The listing builds one solid part. Answer for the finished solid, in the listing's coordinates (mm). Give positions to 0.01 mm unless a question says otherwise; leave off trailing zeros. Loops run counter-clockwise (first coordinate to the right, second up) from the corner with the lowest first, then second, coordinate; pieces in that order, holes last. Notation, with made-up numbers: M 57,31 L 74,31 A12 ccw 74,54 Z; hole C -1,-36.75 d2. An arc over 180 degrees is marked long. Use one line per item in the form item = value. Start each with the question number.
1. The mould has two halves that part along Z. Classify faces 1 (the face through (46.97, 1.61, 41.86)), 2 (the face through (-1, 2, -43)), 3 (the face through (-1, 0, -1)), 4 (the face through (-40.674, 1.565, 22.616)): released by +Z, released by -Z, zero draft, split by the parting line, or undercut.
2. The part is cut by section C-C (z = -19). Give the number of separate pieces and of enclosed holes in the cut face, and give its area (3 significant figures).
3. The part is cut by section B-B (x = 24). Write down the section's boundary in (y, z) (3 decimals).
4. The part is cut by section A-A (z = -35). Write down the section's boundary in (x, y) (3 decimals).
5. Straight lines are drawn through the part: line 1 (X direction, y = 1.05, z = -35) (3 decimals); line 2 (X direction, y = 2.6, z = -25) (3 decimals); line 3 (X direction, y = 1.45, z = -22.5) (3 decimals). For each, find the intervals that lie inside material, in ascending order. Write a range as from..to.
6. Each of these flat-tipped pins is pushed along its axis until it touches: pin 1 Ø2.5 at (x, z) = (-42.68, -18.67) entering from +Y; pin 2 Ø6.5 at (x, z) = (-42.68, 5.84) entering from +Y (3 decimals). Where does it stop, or does it pass through?
from build123d import *

# Parameters (mm, degrees)
SKETCH1_W           = 96.35
SKETCH1_H           = 86
SKETCH1_R           = 2.05
BOSS_EXTRUDE1_DEPTH = 3.175
FILLET1_R           = 4
SKETCH2_R           = 7.05
CUT_EXTRUDE1_DEPTH  = 3.18


with BuildPart() as part:
    # Sketch1 → Boss-Extrude1 (new body)
    with BuildSketch(Plane(origin=(0, 0, 0), x_dir=(1, 0, 0), z_dir=(0, 1, 0))):
        Rectangle(SKETCH1_W, SKETCH1_H)
        with Locations(Location((42.675, 35, 0), (0, 0, 270))):
            Circle(SKETCH1_R, mode=Mode.SUBTRACT)
        with Locations(Location((42.675, 26.832661921, 0), (0, 0, 270))):
            Circle(SKETCH1_R, mode=Mode.SUBTRACT)
        with Locations(Location((42.675, 18.665323842, 0), (0, 0, 270))):
            Circle(SKETCH1_R, mode=Mode.SUBTRACT)
        with Locations(Location((42.675, 10.497985763, 0), (0, 0, 270))):
            Circle(SKETCH1_R, mode=Mode.SUBTRACT)
        with Locations(Location((42.675, 2.330647684, 0), (0, 0, 270))):
            Circle(SKETCH1_R, mode=Mode.SUBTRACT)
        with Locations(Location((42.675, -5.836690395, 0), (0, 0, 270))):
            Circle(SKETCH1_R, mode=Mode.SUBTRACT)
        with Locations(Location((42.675, -14.004028475, 0), (0, 0, 270))):
            Circle(SKETCH1_R, mode=Mode.SUBTRACT)
        with Locations(Location((42.675, -22.171366554, 0), (0, 0, 270))):
            Circle(SKETCH1_R, mode=Mode.SUBTRACT)
        with Locations(Location((42.675, -30.338704633, 0), (0, 0, 270))):
            Circle(SKETCH1_R, mode=Mode.SUBTRACT)
        with Locations(Location((42.675, -38.506042712, 0), (0, 0, 270))):
            Circle(SKETCH1_R, mode=Mode.SUBTRACT)
        with Locations(Location((-42.675, -38.506042712, 0), (0, 0, 90))):
            Circle(SKETCH1_R, mode=Mode.SUBTRACT)
        with Locations(Location((-42.675, -30.338704633, 0), (0, 0, 90))):
            Circle(SKETCH1_R, mode=Mode.SUBTRACT)
        with Locations(Location((-42.675, -22.171366554, 0), (0, 0, 90))):
            Circle(SKETCH1_R, mode=Mode.SUBTRACT)
        with Locations(Location((-42.675, -14.004028475, 0), (0, 0, 90))):
            Circle(SKETCH1_R, mode=Mode.SUBTRACT)
        with Locations(Location((-42.675, -5.836690395, 0), (0, 0, 90))):
            Circle(SKETCH1_R, mode=Mode.SUBTRACT)
        with Locations(Location((-42.675, 2.330647684, 0), (0, 0, 90))):
            Circle(SKETCH1_R, mode=Mode.SUBTRACT)
        with Locations(Location((-42.675, 10.497985763, 0), (0, 0, 90))):
            Circle(SKETCH1_R, mode=Mode.SUBTRACT)
        with Locations(Location((-42.675, 18.665323842, 0), (0, 0, 90))):
            Circle(SKETCH1_R, mode=Mode.SUBTRACT)
        with Locations(Location((-42.675, 26.832661921, 0), (0, 0, 90))):
            Circle(SKETCH1_R, mode=Mode.SUBTRACT)
        with Locations(Location((-42.675, 35, 0), (0, 0, 90))):
            Circle(SKETCH1_R, mode=Mode.SUBTRACT)
    extrude(amount=BOSS_EXTRUDE1_DEPTH)

    # Fillet1
    fillet1_edges = [part.edges().sort_by_distance(p)[0] for p in [
        (48.175, 1.5875, 43),
        (-48.175, 1.5875, 43),
        (-48.175, 1.5875, -43),
        (48.175, 1.5875, -43),
    ]]
    fillet(fillet1_edges, radius=FILLET1_R)

    # Sketch2 → Cut-Extrude1 (cut)
    with BuildSketch(Plane(origin=(0, 3.175, 0), x_dir=(1, 0, 0), z_dir=(0, 1, 0))):
        with Locations(Location((-24, 19, 0), (0, 0, 270))):
            Circle(SKETCH2_R)
        with Locations(Location((24, 19, 0), (0, 0, 270))):
            Circle(SKETCH2_R)
    extrude(amount=-CUT_EXTRUDE1_DEPTH, mode=Mode.SUBTRACT)


solid = part.part
Derived:
q1.face_1 = released by +Z
q1.face_2 = released by -Z
q1.face_3 = zero draft
q1.face_4 = undercut
q2.separate_pieces = 5
q2.enclosed_holes = 0
q2.area = 191 mm2
q3.outline = M 0,-43 L 3.175,-43 L 3.175,-26.05 L 0,-26.05 Z; M 0,-11.95 L 3.175,-11.95 L 3.175,43 L 0,43 Z
q4.outline = M -48.175,0 L -44.725,0 L -44.725,3.175 L -48.175,3.175 Z; M -40.625,0 L 40.625,0 L 40.625,3.175 L -40.625,3.175 Z; M 44.725,0 L 48.175,0 L 48.175,3.175 L 44.725,3.175 Z
q5.line_1 = -48.175..-44.725, -40.625..40.625, 44.725..48.175
q5.line_2 = -48.175..-43.594, -41.756..-27.702, -20.298..20.298, 27.702..41.756, 43.594..48.175
q5.line_3 = -48.175..-30.12, -17.88..17.88, 30.12..48.175
q6.pin_1 = through
q6.pin_2 = 3.175
